Here's how the part is built. I have some questions about the finished solid (model axes, mm). Face numbers are marked on the shaded views. A direction names the side the tool comes from. Round coordinates to 2 decimals unless told otherwise and drop trailing zeros. Loops run counter-clockwise (first coordinate to the right, second up) from the corner with the lowest first, then second, coordinate; pieces in that order, holes last. Notation, with made-up numbers: M -35,47.5 L -8,47.5 A26 ccw -8,71.5 Z; hole C 75,-1.75 d2. An arc over 180 degrees is marked long. Use a Markdown table: item, result.
from build123d import *

# Parameters (mm, degrees)
SKETCH1_R           = 24.75
BOSS_EXTRUDE1_DEPTH = 59.5
SKETCH2_R           = 4
BOSS_EXTRUDE2_DEPTH = 26
CHAMFER1_SIZE       = 3.81
CHAMFER2_SIZE       = 3.81
SKETCH3_R           = 2.25
CUT_EXTRUDE3_DEPTH  = 12.7


with BuildPart() as part:
    # Sketch1 → Boss-Extrude1 (new body)
    with BuildSketch(Plane.XY):
        Circle(SKETCH1_R)
    extrude(amount=BOSS_EXTRUDE1_DEPTH)

    # Sketch2 → Boss-Extrude2 (add)
    with BuildSketch(Plane.XY.offset(59.5)):
        with Locations(Location((0, 0, 0), (0, 0, 180))):
            Circle(SKETCH2_R)
    extrude(amount=BOSS_EXTRUDE2_DEPTH)

    # Chamfer1
    chamfer1_edges = [part.edges().sort_by_distance(p)[0] for p in [
        (-24.75, 0, 59.5),
    ]]
    chamfer(chamfer1_edges, length=CHAMFER1_SIZE)

    # Chamfer2
    chamfer2_edges = [part.edges().sort_by_distance(p)[0] for p in [
        (-24.75, 0, 0),
    ]]
    chamfer(chamfer2_edges, length=CHAMFER2_SIZE)

    # Sketch3 → Cut-Extrude3 (cut)
    with BuildSketch(Plane.XY.offset(59.5)):
        with Locations((0, 15)):
            Circle(SKETCH3_R)
        with Locations((15, 0)):
            Circle(SKETCH3_R)
        with Locations((0, -15)):
            Circle(SKETCH3_R)
        with Locations((-15, 0)):
            Circle(SKETCH3_R)
    extrude(amount=-CUT_EXTRUDE3_DEPTH, mode=Mode.SUBTRACT)


solid = part.part
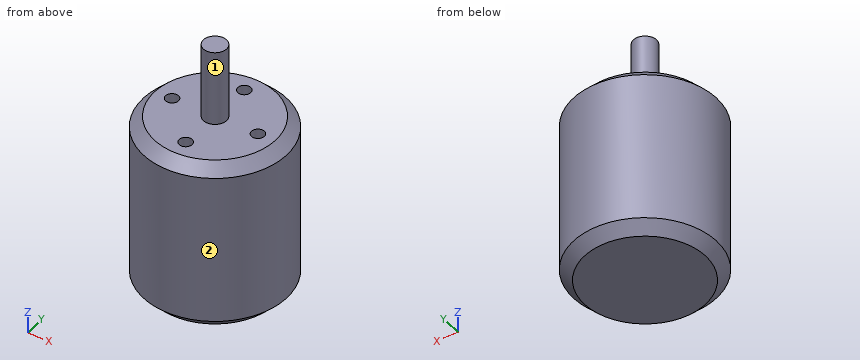
1. Which directions (+Z, -Z, +X, -X, +Y, -Y) give clear straight access to the entire face, cutting with the end or side of a thin tool? Please do the marked faces 1 and 2.
Answer sheet:
| item | result |
|---|---|
| face 1 | +Z |
| face 2 | +Z, -Z |
2. For pin 1 Ø2.5 at (x, y) = (0, 15) entering from +Z; pin 2 Ø8 at (x, z) = (-9.5, 33) entering from +Y; pin 3 Ø5 at (y, z) = (-10, 63) entering from +X; pin 4 Ø3.5 at (x, y) = (15.5, 0.5) entering from +Z, each with a flat end and sliding along its axis, tell me the tip position at first contact or that it passes through.
Answer sheet:
| item | result |
|---|---|
| pin 1 | z = 46.8 |
| pin 2 | y = 24.13 |
| pin 3 | through |
| pin 4 | z = 59.5 |
3. Imagine slicing it at A-A, the plane y = 0. Write out the boundary of the cut face in (x, z), then the cut area to 3 significant figures.
Answer sheet:
| item | result |
|---|---|
| outline | M -24.75,3.81 L -20.94,0 L 20.94,0 L 24.75,3.81 L 24.75,55.69 L 20.94,59.5 L 17.25,59.5 L 17.25,46.8 L 12.75,46.8 L 12.75,59.5 L 4,59.5 L 4,85.5 L -4,85.5 L -4,59.5 L -12.75,59.5 L -12.75,46.8 L -17.25,46.8 L -17.25,59.5 L -20.94,59.5 L -24.75,55.69 Z |
| area | 3,010 mm2 |
4. Imagine slicing it at C-C, the plane z = 15. Write out the boundary of the cut face in (x, y).
Answer sheet:
| item | result |
|---|---|
| outline | C 0,0 d49.5 |
5. I need wall thicknesses on probe 1 along Y at (x, z) = (0, 56); probe 2 along Z at (x, y) = (3, -4); probe 3 along Y at (x, z) = (-15, 50.5). Which ranges of each line are inside material? Lowest first, please. Write a range as from..to.
Answer sheet:
| item | result |
|---|---|
| probe 1 | -24.44..-17.25, -12.75..12.75, 17.25..24.44 |
| probe 2 | 0..59.5 |
| probe 3 | -19.69..-2.25, 2.25..19.69 |
6. Imagine slicing it at B-B, the plane z = 70. Write out the boundary of the cut face in (x, y), then the cut area to 3 significant figures.
Answer sheet:
| item | result |
|---|---|
| outline | C 0,0 d8 |
| area | 50.3 mm2 |
